Check sheet for the modelled part. Datum: model origin and axes. Units: mm. Give positions to 0.01 mm unless a question says otherwise; leave off trailing zeros. Order: outer loops, then holes, each group sorted by start corner. A loop starts at its lowest first (then second) coordinate and runs counter-clockwise, first axis right, second up.
```python
from build123d import *

# Parameters (mm, degrees)
AXIAL_PROFILE_MM_W     = 8
AXIAL_PROFILE_MM_H     = 31.05
AXIAL_HOLES_DEPTH      = 165.078060691
AXIAL_HOLES_DEPTH_BACK = 165.078060691
SKETCH2_R              = 2.4
SKETCH2_R_2            = 1.65
CUT_EXTRUDE2_START     = 148.7
SKETCH3_R              = 1.25
CUT_EXTRUDE2_DEPTH     = 6


with BuildPart() as part:
    # Axial profile (mm) → Full revolution (revolve)
    with BuildSketch(Plane.XY, mode=Mode.PRIVATE) as full_revolution_sk:
        with Locations((152.7, 18.875)):
            Rectangle(AXIAL_PROFILE_MM_W, AXIAL_PROFILE_MM_H)
    revolve(full_revolution_sk.sketch.rotate(Axis((-110, 0, 0), (1, 0, 0)), 90), axis=Axis((-110, 0, 0), (1, 0, 0)))

    # Sketch2 → Axial holes (cut, two sides: drawn at the far end of the back side and taken through both)
    with BuildSketch(Plane(origin=(0, 0, 0), x_dir=(0, 0, -1), z_dir=(1, 0, 0)).offset(-AXIAL_HOLES_DEPTH_BACK)):
        with Locations((-1.977382665, 12.848733704)):
            Circle(SKETCH2_R)
        with Locations((-7.687206041, 10.483647423)):
            Circle(SKETCH2_R)
        with Locations((-29.4, 0)):
            Circle(SKETCH2_R_2)
        with Locations((14.7, -25.461146871)):
            Circle(SKETCH2_R_2)
        with Locations((14.7, 25.461146871)):
            Circle(SKETCH2_R_2)
    extrude(amount=AXIAL_HOLES_DEPTH + AXIAL_HOLES_DEPTH_BACK, mode=Mode.SUBTRACT)

    # Sketch3 → Cut-Extrude2 (cut)
    with BuildSketch(Plane(origin=(0, 0, 0), x_dir=(0, 0, -1), z_dir=(1, 0, 0)).offset(CUT_EXTRUDE2_START)):
        with Locations((-12, 0)):
            Circle(SKETCH3_R)
        with Locations((6, -10.392304845)):
            Circle(SKETCH3_R)
        with Locations((6, 10.392304845)):
            Circle(SKETCH3_R)
    extrude(amount=CUT_EXTRUDE2_DEPTH, mode=Mode.SUBTRACT)


solid = part.part
```
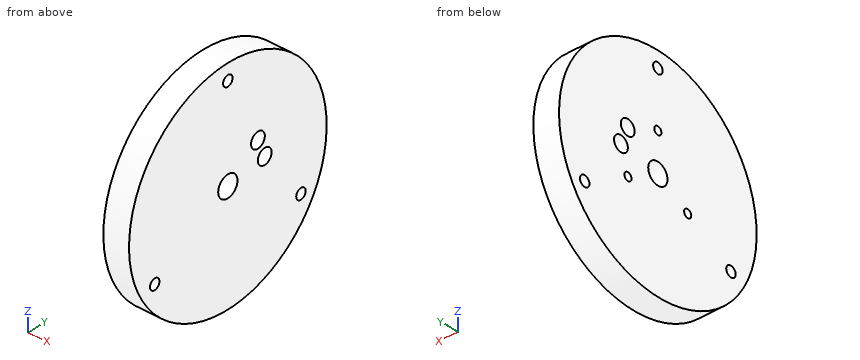
Q1. Sectioned sample at C-C, the plane z = 29.4. Record the cut outline in (x, y), plus the area to 3 significant figures.
Q2. Material ranges on line 1 (Z direction, x = 152.5, y = -1); line 2 (Y direction, x = 151, z = -16); line 3 (Y direction, x = 154.75, z = -14.7), recorded low to high.
Q3. Sectioned sample at B-B, the plane z = -14.7. Record the cut outline in (x, y).
Q4. Go/stop test with flat-tipped pins: P1, Ø4, axis at x = 150.5, z = 5.5, coming from the -Y side; P2, Ø2, axis at y = 25.46, z = -14.7, coming from the +X side; P3, Ø0.8, axis at y = 10.5, z = -6, coming from the -X side; P4, Ø3, axis at x = 153.5, y = -6.5, coming from the +Z side. Record where each tip stops, or that it passes through.
Q5. Sectioned sample at A-A, the plane y = 0. Record the cut outline in (x, z), plus the area to 3 significant figures.
Q6. Sectioned sample at D-D, the plane x = 150. Count the separate pieces of the cut face and the enclosed holes in it, plus the area to 3 significant figures.
Filled in:
1. outline: (148.7, -17.86) - (156.7, -17.86) - (156.7, -1.65) - (148.7, -1.65) - close; (148.7, 1.65) - (156.7, 1.65) - (156.7, 17.86) - (148.7, 17.86) - close
1. area: 259 mm2
2. line 1: z = -34.39 to -3.2, 3.2 to 11.25, 12.75 to 28.09, 30.71 to 34.39
2. line 2: y = -30.45 to -26.48, -24.45 to 24.45, 26.48 to 30.45
2. line 3: y = -31.1 to -27.11, -23.81 to 23.81, 27.11 to 31.1
3. outline: (148.7, -31.1) - (156.7, -31.1) - (156.7, -27.11) - (148.7, -27.11) - close; (148.7, -23.81) - (156.7, -23.81) - (156.7, 23.81) - (148.7, 23.81) - close; (148.7, 27.11) - (156.7, 27.11) - (156.7, 31.1) - (148.7, 31.1) - close
4. P1: stops at y = -34.22
4. P2: passes through
4. P3: stops at x = 154.7
4. P4: stops at z = 34.03
5. outline: (148.7, -34.4) - (156.7, -34.4) - (156.7, -3.35) - (148.7, -3.35) - close; (148.7, 3.35) - (156.7, 3.35) - (156.7, 27.75) - (148.7, 27.75) - (148.7, 13.25) - (154.7, 13.25) - (154.7, 10.75) - (148.7, 10.75) - close; (148.7, 31.05) - (156.7, 31.05) - (156.7, 34.4) - (148.7, 34.4) - close
5. area: 455 mm2
6. separate pieces: 1
6. enclosed holes: 9
6. area: 3,610 mm2
